Here's how the part is built. I have some questions about the finished solid (model axes, mm). Face numbers are marked on the shaded views. A direction names the side the tool comes from. Round coordinates to 2 decimals unless told otherwise and drop trailing zeros. Loops run counter-clockwise (first coordinate to the right, second up) from the corner with the lowest first, then second, coordinate; pieces in that order, holes last. Notation, with made-up numbers: M 19,42.25 L 44,42.25 A22 ccw 44,63.25 Z; hole C 24.25,-38 d2. An arc over 180 degrees is marked long. Answer as a JSON object with one key per item and string values.
from build123d import *

# Parameters (mm, degrees)
F0_W     = 15.9
F0_H     = 15.9
F0_R     = 2.45
F1_DEPTH = 9.5
F2_DEPTH = 11.4
F3_R     = 2.725
F5_DEPTH = 9.5
F6_DEPTH = 25
F7_T     = -1.5


with BuildPart() as f1:
    # F0 (on Top) → F1 (new body)
    with BuildSketch(Plane.XY):
        with Locations((7.95, -7.95)):
            Rectangle(F0_W, F0_H)
        with Locations((3.95, -11.95)):
            Circle(F0_R, mode=Mode.SUBTRACT)
        with Locations((3.95, -3.95)):
            Circle(F0_R, mode=Mode.SUBTRACT)
    extrude(amount=F1_DEPTH)

    # F0 (on Top) → F2 (join)
    with BuildSketch(Plane.XY):
        with Locations((3.95, -3.95)):
            Circle(F0_R)
        with Locations((3.95, -11.95)):
            Circle(F0_R)
    extrude(amount=F2_DEPTH)

    # F3 (on face) → F5 (join)
    with BuildSketch(Plane.XY):
        with BuildLine():
            ThreePointArc((5.8339274183, -5.5163069567), (5.6824116139, -5.6824116139), (5.5163069567, -5.8339274183))
            ThreePointArc((5.5163069567, -5.8339274183), (4.725, -7.95), (5.5163069567, -10.0660725817))
            ThreePointArc((5.5163069567, -10.0660725817), (5.6824116139, -10.2175883861), (5.8339274183, -10.3836930433))
            ThreePointArc((5.8339274183, -10.3836930433), (9.287215563, -10.884702632), (11.175, -7.95))
            ThreePointArc((11.175, -7.95), (9.287215563, -5.015297368), (5.8339274183, -5.5163069567))
        make_face()
        with Locations((7.95, -7.95)):
            Circle(F3_R, mode=Mode.SUBTRACT)
    extrude(amount=F5_DEPTH)

    # F4 (on face) → F6 (cut)
    with BuildSketch(Plane.XZ.offset(15.9)):
        Polygon((15.9, 9.5), (7.95, 9.5), (15.9, 0), align=None)
    extrude(amount=-F6_DEPTH, mode=Mode.SUBTRACT)

    # F7
    f7_openings = [f1.faces().sort_by_distance(p)[0] for p in [
        (7.95, -7.95, 0),
    ]]
    offset(amount=F7_T, openings=f7_openings, kind=Kind.INTERSECTION)


solid = f1.part
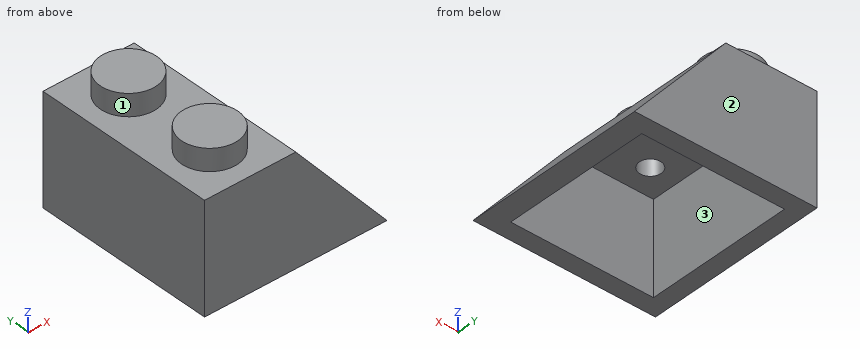
Item 1: For the marked faces 1, 2 and 3, which set-ups out of +Z, -Z, +X, -X, +Y, -Y let a thin tool reach every point of the face, with its end or its side?
Solution:
{"face 1": "+Z", "face 2": "+Z, -Z, +X, -X, +Y", "face 3": "-Z"}
Item 2: For P1, Ø4, axis at y = -13.5, z = 8, coming from the +X side; P2, Ø2.5, axis at x = 3.5, y = -7.5, coming from the +Z side; P3, Ø4.5, axis at x = 4.5, y = -7, coming from the -Z side; P4, Ø5, axis at x = 11, y = -8, coming from the -Z side, each with a flat end and sliding along its axis, tell me the tip position at first contact or that it passes through.
Solution:
{"P1": "stops at x = 10.88", "P2": "stops at z = 11.4", "P3": "stops at z = 8", "P4": "stops at z = 0.53"}
Item 3: I want a section at B-B on x = 3.95. List the corners of the cut face in (y, z) for me.
Solution:
{"outline": "M -15.9,0 L -14.4,0 L -14.4,8 L -12.9,8 L -12.9,9.9 L -11,9.9 L -11,8 L -4.9,8 L -4.9,9.9 L -3,9.9 L -3,8 L -1.5,8 L -1.5,0 L 0,0 L 0,9.5 L -1.5,9.5 L -1.5,11.4 L -6.4,11.4 L -6.4,9.5 L -9.5,9.5 L -9.5,11.4 L -14.4,11.4 L -14.4,9.5 L -15.9,9.5 Z"}
Item 4: I want a section at C-C on z = 9.25. List the corners of the cut face in (x, y) for me.
Solution:
{"outline": "M 0,-15.9 L 8.16,-15.9 L 8.16,0 L 0,0 Z; hole C 3.95,-11.95 d1.9; hole C 3.95,-3.95 d1.9"}
Item 5: If I drill on L1, parallel to Y at x = 3.95, z = 9; L2, parallel to Y at x = 4, z = 6; L3, parallel to X at y = -3.95, z = 8.65, over which ranges is the centre line in solid material (lowest first)? Write a range as from..to.
Solution:
{"L1": "y = -15.9..-12.9, -11..-4.9, -3..0", "L2": "y = -15.9..-14.4, -1.5..0", "L3": "x = 0..3, 4.9..8.66"}
Item 6: I want a section at A-A on y = -3.95. List the corners of the cut face in (x, z) for me.
Solution:
{"outline": "M 0,0 L 1.5,0 L 1.5,8 L 3,8 L 3,9.9 L 4.9,9.9 L 4.9,8 L 7.25,8 L 13.94,0 L 15.9,0 L 7.95,9.5 L 6.4,9.5 L 6.4,11.4 L 1.5,11.4 L 1.5,9.5 L 0,9.5 Z"}
Item 7: I want a section at D-D on z = 5.5. List the corners of the cut face in (x, y) for me, plus the area to 3 significant figures.
Solution:
{"outline": "M 0,-15.9 L 11.3,-15.9 L 11.3,0 L 0,0 Z; hole M 1.5,-14.4 L 9.34,-14.4 L 9.34,-1.5 L 1.5,-1.5 Z", "area": "78.5 mm2"}
